Read the model definition and answer for the solid it produces. Units are mm, in the model's axes. Face numbers are marked on the shaded views. A direction names the side the tool comes from. Round coordinates to 2 decimals unless told otherwise and drop trailing zeros. Write each loop counter-clockwise with the first axis right and the second up, starting at its lowest first coordinate (ties: lowest second). Pieces come first, ordered by that corner, then holes. Notation, with made-up numbers: (54.25, 64.25) -> (108.25, 64.25) arc R11 ccw to (108.25, 76.25) -> close; hole circle Ø5 at (51, 25.5). An arc over 180 degrees is marked (long way). Return JSON: item names as keys, results as strings.
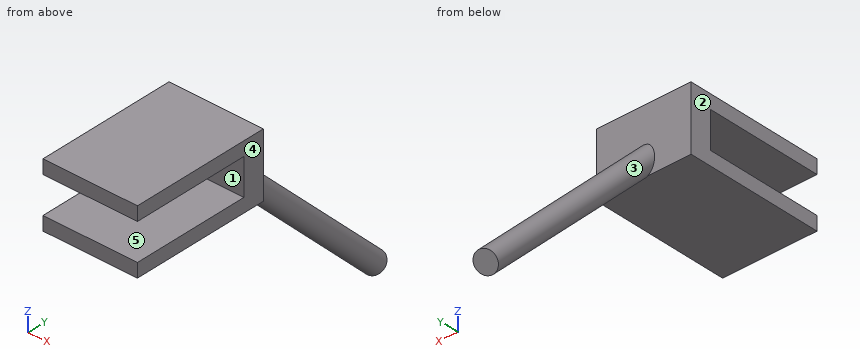
from build123d import *

# Parameters (mm, degrees)
SKETCH1_W               = 44
SKETCH1_H               = 30
BOSS_EXTRUDE1_DEPTH     = 65
CUT_EXTRUDE1_DEPTH      = 80.912452096
CUT_EXTRUDE1_DEPTH_BACK = 80.912452096
SKETCH2_W               = 17
SKETCH2_H               = 55
SKETCH3_R               = 5
BOSS_EXTRUDE2_DEPTH     = 120
SKETCH3_2_R             = 5
BOSS_EXTRUDE3_DEPTH     = 120


with BuildPart() as part:
    # Sketch1 → Boss-Extrude1 (new body)
    with BuildSketch(Plane(origin=(0, 0, 0), x_dir=(1, 0, 0), z_dir=(0, 1, 0))):
        Rectangle(SKETCH1_W, SKETCH1_H)
    extrude(amount=BOSS_EXTRUDE1_DEPTH)

    # Sketch2 → Cut-Extrude1 (cut, two sides: drawn at the far end of the back side and taken through both)
    with BuildSketch(Plane(origin=(22, 0, 0), x_dir=(0, 0, -1), z_dir=(1, 0, 0)).offset(-CUT_EXTRUDE1_DEPTH_BACK)):
        with Locations((0, 27.5)):
            Rectangle(SKETCH2_W, SKETCH2_H)
    extrude(amount=CUT_EXTRUDE1_DEPTH + CUT_EXTRUDE1_DEPTH_BACK, mode=Mode.SUBTRACT)

    # Sketch3 → Boss-Extrude2 (add)
    with BuildSketch(Plane(origin=(0, 33.487457391, -33.487457391), x_dir=(8.429181601007666e-15, -0.7071067811865441, -0.707106781186551), z_dir=(-8.648297214624002e-15, 0.707106781186551, -0.7071067811865441))):
        with Locations(Location((-40, 0, 0), (0, 0, 21.731030202))):
            Circle(SKETCH3_R)
    extrude(amount=BOSS_EXTRUDE2_DEPTH)

    # Sketch3_2 → Boss-Extrude3 (add)
    with BuildSketch(Plane(origin=(0, 33.487457391, -33.487457391), x_dir=(8.429181601007666e-15, -0.7071067811865441, -0.707106781186551), z_dir=(-8.648297214624002e-15, 0.707106781186551, -0.7071067811865441))):
        with Locations(Location((-40, 0, 0), (0, 0, 21.731030202))):
            Circle(SKETCH3_2_R)
    extrude(amount=BOSS_EXTRUDE3_DEPTH)


solid = part.part
Item 1: Flat-ended cylindrical pins translate along their axes: pin 1 (22 mm diameter, centred on x = 5.5, y = 28.5, fed in from -Z); pin 2 (9 mm diameter, centred on x = -4.5, z = -5.5, fed in from +Y); pin 3 (8.5 mm diameter, centred on x = -8, z = 0, fed in from -Y). Find the tip coordinate at first contact, or state that the pin passes through.
Worked answers:
{"pin 1": "stops at z = -15", "pin 2": "stops at y = 72.29", "pin 3": "stops at y = 55"}
Item 2: For a pull along Z with two mould halves and no side action, classify the marked faces 3, 4 and 5 as released by +Z, released by -Z, zero draft, split by the parting line, or undercut.
Worked answers:
{"face 3": "split by the parting line", "face 4": "zero draft", "face 5": "undercut"}
Item 3: Section C-C (y = 60) is taken. Give the vertices of the cut face in (x, z), then the cut area to 3 significant figures.
Worked answers:
{"outline": "(-22, -15) -> (22, -15) -> (22, 15) -> (-22, 15) -> close", "area": "1,320 mm2"}
Item 4: A tool of negligible diameter and unlimited length cuts with its end or side. For the marked faces 1 and 2, from which of +Z, -Z, +X, -X, +Y, -Y can it reach the whole face along a straight path? Write none if from no direction.
Worked answers:
{"face 1": "+X, -X, -Y", "face 2": "+Z, -Z, -X, +Y, -Y"}
Item 5: Straight lines are drawn through the part: L1, parallel to Z at x = -14.5, y = 40; L2, parallel to Y at x = -18, z = 10; L3, parallel to Z at x = -4, y = 57. For each, find the intervals that lie inside material, in ascending order. Write a range as [from, to].
Worked answers:
{"L1": "z = [-15, -8.5], [8.5, 15]", "L2": "y = [0, 65]", "L3": "z = [-15, 15]"}
Item 6: Section A-A (y = 18.5) is taken. Give the vertices of the cut face in (x, z), then the cut area to 3 significant figures.
Worked answers:
{"outline": "(-22, -15) -> (22, -15) -> (22, -8.5) -> (-22, -8.5) -> close; (-22, 8.5) -> (22, 8.5) -> (22, 15) -> (-22, 15) -> close", "area": "572 mm2"}
Item 7: Section D-D (x = -19) is taken. Give the vertices of the cut face in (y, z), then the cut area to 4 significant figures.
Worked answers:
{"outline": "(0, -15) -> (65, -15) -> (65, 15) -> (0, 15) -> (0, 8.5) -> (55, 8.5) -> (55, -8.5) -> (0, -8.5) -> close", "area": "1,015 mm2"}
Item 8: Section B-B (x = 0) is taken. Give the vertices of the cut face in (y, z), then the cut area to 3 significant figures.
Worked answers:
{"outline": "(0, -15) -> (64.5, -15) -> (143.09, -93.59) -> (150.16, -86.52) -> (65.31, -1.67) -> (65, -1.97) -> (65, 15) -> (0, 15) -> (0, 8.5) -> (55, 8.5) -> (55, -8.5) -> (0, -8.5) -> close", "area": "2,170 mm2"}
